Part print with two shaded views. Sizes in mm from the minimum x, y, z corner. A direction names the side the tool comes from. Coordinates: 2 decimals unless noted, no trailing zeros. Order: outer loops, then holes, each group sorted by start corner. A loop starts at its lowest first (then second) coordinate and runs counter-clockwise, first axis right, second up. Notation, with made-up numbers: (72.25, 81) - (91.25, 81) arc R25 ccw to (91.25, 105) - close; hole circle Ø5 at (73.25, 55.5). An arc over 180 degrees is marked (long way). Write each question's results on one line, items separated by ' | '. Start each with the question number.
Q1. Which spindle directions (+Z, -Z, +X, -X, +Y, -Y) get a long thin tool onto all of the face, cutting with end or side? Do the marked faces 1, 2 and 3. Say none if no direction does.
Q2. Band-saw the part on C-C, the plane z = 24. Write the cut outline in (x, y) (3 decimals), then the cut area to 3 significant figures.
Q3. Band-saw the part on B-B, the plane x = 87.5. Count the separate pieces of the cut face and the enclosed holes in it, then the cut area to 3 significant figures.
Q4. Pull direction Z, two halves, no side cores. Call the marked faces 4, 5 and 6: released by +Z, released by -Z, zero draft, split by the parting line, or undercut.
Q5. Pin check, flat tips, straight feed: P1, Ø4, axis at y = 16, z = 22.5, coming from the -X side (3 decimals); P2, Ø4, axis at y = 9, z = 8, coming from the -X side; P3, Ø1, axis at y = 5, z = 26.5, coming from the +X side; P4, Ø7.5, axis at x = 92.075, y = 15.875, coming from the -Z side. Stop position of each tip, or through.
Q6. Wall check: probe 1 along Y at (x, z) = (11, 10) (3 decimals); probe 2 along X at (y, z) = (8, 15.5). Give the ranges that are in metal, low to high.
Q7. Band-saw the part on A-A, the plane x = 76.5. Write the cut outline in (y, z) (3 decimals), then the cut area to 3 significant figures.
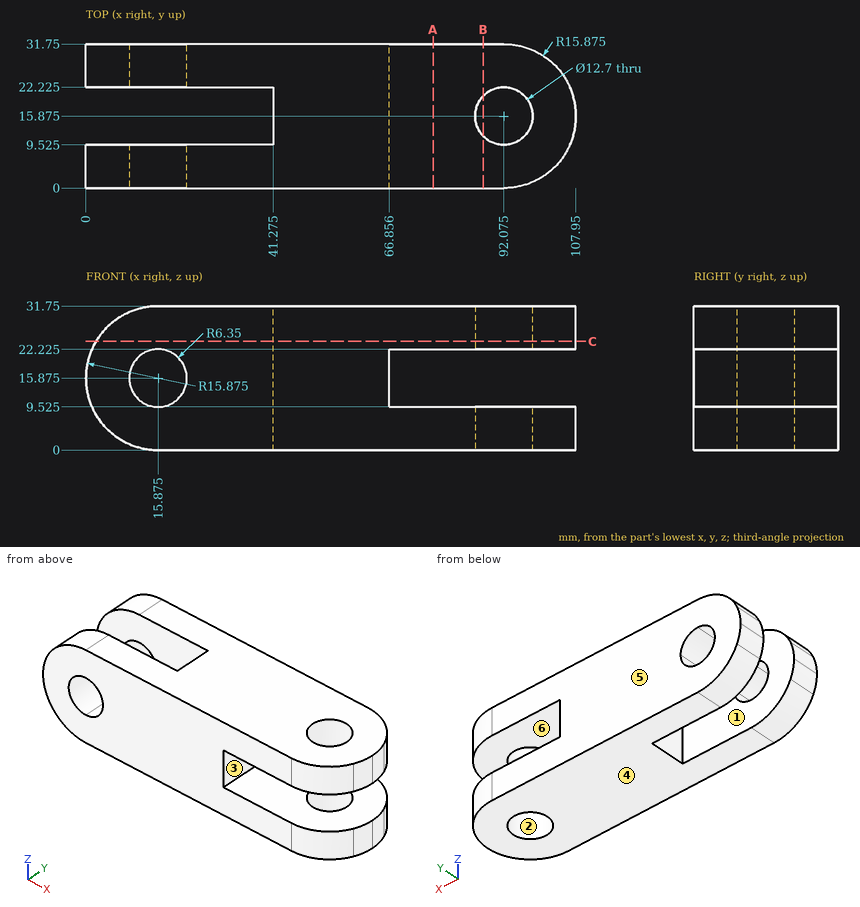
Results below:
1) face 1: +Z, -Z, -X | face 2: +Z, -Z | face 3: +X, +Y, -Y
2) outline: (2.237, 0) - (92.075, 0) arc R15.875 ccw to (92.075, 31.75) - (2.237, 31.75) - (2.237, 22.225) - (41.275, 22.225) - (41.275, 9.525) - (2.237, 9.525) - close; hole circle Ø12.7 at (92.075, 15.875) | area: 2,630 mm²
3) separate pieces: 4 | enclosed holes: 0 | area: 437 mm²
4) face 4: released by -Z | face 5: zero draft | face 6: undercut
5) P1: stops at x = 41.275 | P2: stops at x = 1.13 | P3: stops at x = 104.09 | P4: passes through
6) probe 1: y = 0 to 9.525, 22.225 to 31.75 | probe 2: x = 0 to 9.54, 22.21 to 66.86
7) outline: (0, 0) - (31.75, 0) - (31.75, 9.525) - (0, 9.525) - close; (0, 22.225) - (31.75, 22.225) - (31.75, 31.75) - (0, 31.75) - close | area: 605 mm²
